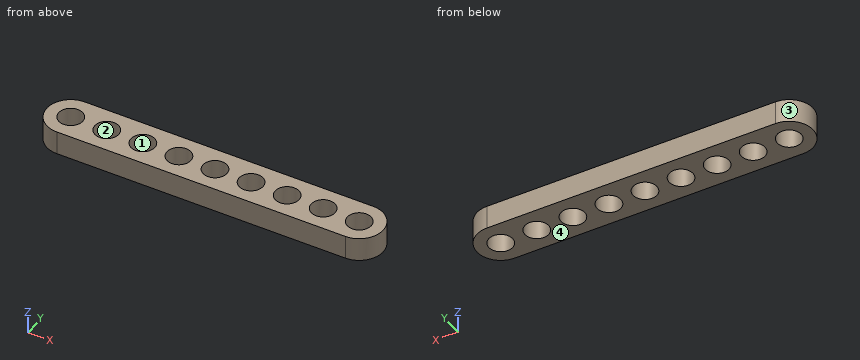
from build123d import *

# Parameters (mm, degrees)
SKETCH1_R           = 5
BOSS_EXTRUDE1_DEPTH = 10


with BuildPart() as part:
    # Sketch1 → Boss-Extrude1 (new body)
    with BuildSketch(Plane.XY):
        with BuildLine():
            Line((-60, 10), (60, 10))
            ThreePointArc((60, 10), (70, 0), (60, -10))
            Line((60, -10), (-60, -10))
            ThreePointArc((-60, -10), (-70, 0), (-60, 10))
        make_face()
        with Locations((-60, 0)):
            Circle(SKETCH1_R, mode=Mode.SUBTRACT)
        with Locations((-45, 0)):
            Circle(SKETCH1_R, mode=Mode.SUBTRACT)
        with Locations((-30, 0)):
            Circle(SKETCH1_R, mode=Mode.SUBTRACT)
        with Locations((-15, 0)):
            Circle(SKETCH1_R, mode=Mode.SUBTRACT)
        Circle(SKETCH1_R, mode=Mode.SUBTRACT)
        with Locations((15, 0)):
            Circle(SKETCH1_R, mode=Mode.SUBTRACT)
        with Locations((30, 0)):
            Circle(SKETCH1_R, mode=Mode.SUBTRACT)
        with Locations((45, 0)):
            Circle(SKETCH1_R, mode=Mode.SUBTRACT)
        with Locations((60, 0)):
            Circle(SKETCH1_R, mode=Mode.SUBTRACT)
    extrude(amount=BOSS_EXTRUDE1_DEPTH)


solid = part.part
Geometry check sheet. Reference: the model listing, model coordinates, mm. Face numbers are marked on the shaded views. Round coordinates to 2 decimals unless told otherwise and drop trailing zeros. Order: outer loops, then holes, each group sorted by start corner. A loop starts at its lowest first (then second) coordinate and runs counter-clockwise, first axis right, second up. Notation, with made-up numbers: M 71.25,-0.75 L 77.25,-0.75 A32 ccw 77.25,32.25 Z; hole C 83.5,75 d6. An arc over 180 degrees is marked long. Write each question's results on one line, items separated by ' | '. Start each with the question number.
1. Cross-section at A-A on x = 45. Record the boundary of the cut face in (y, z).
2. Cross-section at D-D on x = 2. Record the boundary of the cut face in (y, z).
3. Cross-section at B-B on z = 5.5. Give the number of separate pieces and of enclosed holes in the cut face, plus the area to 3 significant figures.
4. Draft check along X on the marked faces 1, 2, 3 and 4. Enter one of: pulls with the +X half, pulls with the -X half, needs draft (parallel to the pull), parting line crosses it, or undercut.
5. Material ranges on L1, parallel to Y at x = 60, z = 5; L2, parallel to Y at x = -3.5, z = 5; L3, parallel to X at y = -7, z = 6.5, recorded low to high. Write a range as from..to.
Resolved:
1) outline: M -10,0 L -5,0 L -5,10 L -10,10 Z; M 5,0 L 10,0 L 10,10 L 5,10 Z
2) outline: M -10,0 L -4.58,0 L -4.58,10 L -10,10 Z; M 4.58,0 L 10,0 L 10,10 L 4.58,10 Z
3) separate pieces: 1 | enclosed holes: 9 | area: 2,010 mm2
4) face 1: undercut | face 2: undercut | face 3: pulls with the -X half | face 4: needs draft
5) L1: -10..-5, 5..10 | L2: -10..-3.57, 3.57..10 | L3: -67.14..67.14
